For this review, take the finished solid that the model builds, in its own axes (mm). Face numbers are marked on the shaded views. A direction names the side the tool comes from. Give positions to 0.01 mm unless a question says otherwise; leave off trailing zeros. Order: outer loops, then holes, each group sorted by start corner. A loop starts at its lowest first (then second) coordinate and runs counter-clockwise, first axis right, second up. Notation, with made-up numbers: (26, 22) -> (41, 22) arc R6 ccw to (41, 27) -> close; hole circle Ø8 at (72, 78.25). An arc over 180 degrees is marked (long way). Return JSON: item names as keys, results as strings. Group by question number.
1) To check wall thickness, follow line 1 along X through (y, z) = (2, -74); line 2 along X through (y, z) = (9.3, -6); line 3 along Z through (x, y) = (73, 3.5). State the ranges of each line that lie inside material, in increasing order.
2) Add section A-A (z = -45). Give the boundary of the cut face in (x, y), then the cut area to 3 significant figures.
3) The part is to be moulded in two halves that separate along Z. For the marked faces 3, 4, 5 and 6, say which applies: released by +Z, released by -Z, zero draft, split by the parting line, or undercut.
4) Insertion check: P1, Ø7, axis at x = 25, z = -45, coming from the -Y side; P2, Ø2.5, axis at x = 105, z = -6, coming from the +Y side; P3, Ø6, axis at x = 6, z = -6, coming from the -Y side. Each pin has a flat end and moves straight along its axis. Give the tip position at first contact, or say it passes through.
5) Add section C-C (x = 69.5). Give the boundary of the cut face in (y, z), then the cut area to 3 significant figures.
6) Add section D-D (z = -59.5). Give the boundary of the cut face in (x, y).
7) Add section B-B (y = 4.25). State how many separate pieces and enclosed holes the cut face has, then the cut area to 3 significant figures.
8) For the marked faces 1 and 2, list the 3-axis set-ups (+Z, -Z, +X, -X, +Y, -Y) from which the entire face can be reached by the end or side of a thin tool; tool diameter is ignored.
from build123d import *

# Parameters (mm, degrees)
SKETCH1_W            = 110
SKETCH1_H            = 90
BOSS_EXTRUDE1_DEPTH  = 10
SHELL2_T             = -2
FILLET3_R            = 5
FILLET4_R            = 5
SKETCH5_R            = 4
BOSS_EXTRUDE12_DEPTH = 8
FILLET5_R            = 5
FILLET6_DEPTH        = 9
FILLET7_R            = 5
FILLET8_R            = 5
FILLET9_R            = 5
FILLET10_R           = 5
FILLET11_DEPTH       = 9
FILLET12_DEPTH       = 9
SKETCH6_R            = 1.6
CUT_EXTRUDE1_DEPTH   = 10
SKETCH7_R            = 4
BOSS_EXTRUDE13_DEPTH = 10
SKETCH8_R            = 1.5
CUT_EXTRUDE2_DEPTH   = 8
SKETCH9_R            = 2.75
CUT_EXTRUDE3_DEPTH   = 10
SKETCH10_R           = 2
CUT_EXTRUDE7_DEPTH   = 10
SKETCH11_R           = 2.5
CUT_EXTRUDE8_DEPTH   = 2


with BuildPart() as part:
    # Sketch1 → Boss-Extrude1 (new body)
    with BuildSketch(Plane(origin=(0, 0, 0), x_dir=(1, 0, 0), z_dir=(0, 1, 0))):
        with Locations((55, 45)):
            Rectangle(SKETCH1_W, SKETCH1_H)
    extrude(amount=BOSS_EXTRUDE1_DEPTH)

    # Shell2
    shell2_openings = [part.faces().sort_by_distance(p)[0] for p in [
        (55, 0, -45),
    ]]
    offset(amount=SHELL2_T, openings=shell2_openings, kind=Kind.INTERSECTION)

    # Fillet3
    fillet3_edges = [part.edges().sort_by_distance(p)[0] for p in [
        (0, 5, -90),
        (110, 5, -90),
        (110, 5, 0),
        (0, 5, 0),
    ]]
    fillet(fillet3_edges, radius=FILLET3_R)

    # Fillet4
    fillet4_edges = [part.edges().sort_by_distance(p)[0] for p in [
        (2, 4, -88),
        (2, 4, -2),
        (108, 4, -2),
        (108, 4, -88),
    ]]
    fillet(fillet4_edges, radius=FILLET4_R)

    # Sketch5 → Boss-Extrude12 (add)
    with BuildSketch(Plane(origin=(0, 8, 0), x_dir=(-1, 0, 0), z_dir=(0, -1, 0))):
        with Locations((-104, 6)):
            Circle(SKETCH5_R)
        with Locations((-104, 84)):
            Circle(SKETCH5_R)
        with Locations((-6, 84)):
            Circle(SKETCH5_R)
        with Locations((-6, 6)):
            Circle(SKETCH5_R)
    extrude(amount=BOSS_EXTRUDE12_DEPTH)

    # Fillet5
    # the kernel refuses this fillet: 5 mm, written as the material it adds along each edge
    with BuildSketch(Plane(origin=(107.972048604, 0, -6.472048604), x_dir=(-0.7834590295976485, 0, -0.621443439857491), z_dir=(0, 1, 0))) as fillet5_piece_1_section:
        with BuildLine():
            CenterArc((9.160403969, -3.547792862), FILLET5_R, 134.800989095, 83.620629792)
            Line((5.243108821, -6.655010061), (4.851379306, -6.965731781))
            ThreePointArc((4.851379306, -6.965731781), (-0.085536357, -0.74172022), (-0.422348831, -0.26762187))
            Line((-0.422348831, -0.26762187), (0.35232323, 0.354779286))
            ThreePointArc((0.35232323, 0.354779286), (2.818585837, -0.661765711), (5.284848444, 0.354779286))
            Line((5.284848444, 0.354779286), (5.637171673, 0))
        make_face()
    fillet5_piece_1 = extrude(amount=29.180673535, mode=Mode.PRIVATE)
    fillet5_piece_1 = split(fillet5_piece_1, bisect_by=Plane(origin=(107.972048604, 10, -6.472048604), z_dir=(0, -1, 0)), keep=Keep.TOP, mode=Mode.PRIVATE)
    add(fillet5_piece_1)

    # Fillet6: read off the stored shape, not the designer's step
    # Fillet6 outline → Fillet6 (add)
    with BuildSketch(Plane(origin=(0, 0, 0), x_dir=(1, 0, 0), z_dir=(0, 1, 0))):
        with BuildLine():
            ThreePointArc((100.02476804, 6.444444444), (98.389061423, 3.273220038), (95.05572809, 2))
            Line((95.05572809, 2), (103, 2))
            ThreePointArc((103, 2), (103.264345398, 2.006992739), (103.527951396, 2.027951396))
            ThreePointArc((103.527951396, 2.027951396), (100.866163882, 3.51422624), (100.02476804, 6.444444444))
        make_face()
    extrude(amount=FILLET6_DEPTH)

    # Fillet7
    # the kernel refuses this fillet: 5 mm, written as the material it adds along each edge
    with BuildSketch(Plane(origin=(107.972048604, 0, -83.527951396), x_dir=(0.0032991627515109216, 0, 0.9999945577477605), z_dir=(0, 1, 0))) as fillet7_piece_1_section:
        with BuildLine():
            CenterArc((8.4557736, -4.999972789), FILLET7_R, 89.810971555, 83.620629792)
            Line((3.488593561, -4.428026585), (2.991875557, -4.370831965))
            ThreePointArc((2.991875557, -4.370831965), (2.264117061, -1.804476076), (-0.060643809, -0.496308703))
            Line((-0.060643809, -0.496308703), (-0.051154492, 0.497376334))
            ThreePointArc((-0.051154492, 0.497376334), (0.52969032, 0.526206725), (8.473918995, 0.499997279))
            Line((8.473918995, 0.499997279), (8.472269414, 0))
        make_face()
    fillet7_piece_1 = extrude(amount=29.180673535, mode=Mode.PRIVATE)
    fillet7_piece_1 = split(fillet7_piece_1, bisect_by=Plane(origin=(107.972048604, 10, -83.527951396), z_dir=(0, -1, 0)), keep=Keep.TOP, mode=Mode.PRIVATE)
    add(fillet7_piece_1)

    # Fillet8
    # the kernel refuses this fillet: 5 mm, written as the material it adds along each edge
    with BuildSketch(Plane(origin=(103.527951396, 0, -87.972048604), x_dir=(-0.6214434398574978, 0, 0.783459029597643), z_dir=(0, 1, 0))) as fillet8_piece_1_section:
        with BuildLine():
            CenterArc((9.160403969, -3.547792862), FILLET8_R, 134.800989095, 83.620629792)
            Line((5.243108821, -6.655010061), (4.851379306, -6.965731781))
            ThreePointArc((4.851379306, -6.965731781), (-0.085536357, -0.74172022), (-0.422348831, -0.26762187))
            Line((-0.422348831, -0.26762187), (0.35232323, 0.354779286))
            ThreePointArc((0.35232323, 0.354779286), (2.818585837, -0.661765711), (5.284848444, 0.354779286))
            Line((5.284848444, 0.354779286), (5.637171673, 0))
        make_face()
    fillet8_piece_1 = extrude(amount=29.180673535, mode=Mode.PRIVATE)
    fillet8_piece_1 = split(fillet8_piece_1, bisect_by=Plane(origin=(103.527951396, 10, -87.972048604), z_dir=(0, -1, 0)), keep=Keep.TOP, mode=Mode.PRIVATE)
    add(fillet8_piece_1)

    # Fillet9
    # the kernel refuses this fillet: 5 mm, written as the material it adds along each edge
    with BuildSketch(Plane(origin=(6.472048604, 29.180673535, -2.027951396), x_dir=(0.9999945577477605, 0, 0.003299162751511756), z_dir=(0, -1, 0))) as fillet9_piece_1_section:
        with BuildLine():
            CenterArc((8.4557736, -4.999972789), FILLET9_R, 89.810971555, 83.620629792)
            Line((3.488593561, -4.428026585), (2.991875557, -4.370831965))
            ThreePointArc((2.991875557, -4.370831965), (2.264117061, -1.804476076), (-0.060643809, -0.496308703))
            Line((-0.060643809, -0.496308703), (-0.051154492, 0.497376334))
            ThreePointArc((-0.051154492, 0.497376334), (0.52969032, 0.526206725), (8.473918995, 0.499997279))
            Line((8.473918995, 0.499997279), (8.472269414, 0))
        make_face()
    fillet9_piece_1 = extrude(amount=29.180673535, mode=Mode.PRIVATE)
    fillet9_piece_1 = split(fillet9_piece_1, bisect_by=Plane(origin=(6.472048604, 10, -2.027951396), z_dir=(0, -1, 0)), keep=Keep.TOP, mode=Mode.PRIVATE)
    add(fillet9_piece_1)

    # Fillet10
    # the kernel refuses this fillet: 5 mm, written as the material it adds along each edge
    with BuildSketch(Plane(origin=(2.027951396, 29.180673535, -6.472048604), x_dir=(0.783459029597646, 0, -0.6214434398574942), z_dir=(0, -1, 0))) as fillet10_piece_1_section:
        with BuildLine():
            CenterArc((9.160403969, -3.547792862), FILLET10_R, 134.800989095, 83.620629792)
            Line((5.243108821, -6.655010061), (4.851379306, -6.965731781))
            ThreePointArc((4.851379306, -6.965731781), (-0.085536357, -0.74172022), (-0.422348831, -0.26762187))
            Line((-0.422348831, -0.26762187), (0.35232323, 0.354779286))
            ThreePointArc((0.35232323, 0.354779286), (2.818585837, -0.661765711), (5.284848444, 0.354779286))
            Line((5.284848444, 0.354779286), (5.637171673, 0))
        make_face()
    fillet10_piece_1 = extrude(amount=29.180673535, mode=Mode.PRIVATE)
    fillet10_piece_1 = split(fillet10_piece_1, bisect_by=Plane(origin=(2.027951396, 10, -6.472048604), z_dir=(0, -1, 0)), keep=Keep.TOP, mode=Mode.PRIVATE)
    add(fillet10_piece_1)

    # Fillet11: read off the stored shape, not the designer's step
    # Fillet11 outline → Fillet11 (add)
    with BuildSketch(Plane(origin=(0, 0, 0), x_dir=(1, 0, 0), z_dir=(0, 1, 0))):
        with BuildLine():
            ThreePointArc((2, 75.05572809), (3.273220038, 78.389061423), (6.444444444, 80.02476804))
            ThreePointArc((6.444444444, 80.02476804), (3.51422624, 80.866163882), (2.027951396, 83.527951396))
            ThreePointArc((2.027951396, 83.527951396), (2.006992739, 83.264345398), (2, 83))
            Line((2, 83), (2, 75.05572809))
        make_face()
    extrude(amount=FILLET11_DEPTH)

    # Fillet12: read off the stored shape, not the designer's step
    # Fillet12 outline → Fillet12 (add)
    with BuildSketch(Plane(origin=(0, 0, 0), x_dir=(1, 0, 0), z_dir=(0, 1, 0))):
        with BuildLine():
            ThreePointArc((9.97523196, 83.555555556), (11.610938577, 86.726779962), (14.94427191, 88))
            Line((14.94427191, 88), (7, 88))
            ThreePointArc((7, 88), (6.735654602, 87.993007261), (6.472048604, 87.972048604))
            ThreePointArc((6.472048604, 87.972048604), (9.133836118, 86.48577376), (9.97523196, 83.555555556))
        make_face()
    extrude(amount=FILLET12_DEPTH)

    # Sketch6 → Cut-Extrude1 (cut)
    with BuildSketch(Plane(origin=(0, 0, 0), x_dir=(-1, 0, 0), z_dir=(0, -1, 0))):
        with Locations(Location((-6, 6, 0), (0, 0, 90))):
            Circle(SKETCH6_R)
        with Locations(Location((-104, 84, 0), (0, 0, 90))):
            Circle(SKETCH6_R)
        with Locations(Location((-104, 6, 0), (0, 0, 90))):
            Circle(SKETCH6_R)
        with Locations(Location((-6, 84, 0), (0, 0, 90))):
            Circle(SKETCH6_R)
    extrude(amount=-CUT_EXTRUDE1_DEPTH, mode=Mode.SUBTRACT)

    # Sketch7 → Boss-Extrude13 (add)
    with BuildSketch(Plane(origin=(0, 8, 0), x_dir=(-1, 0, 0), z_dir=(0, -1, 0))):
        with Locations(Location((-95.5, 15.7, 0), (0, 0, 90))):
            Circle(SKETCH7_R)
        with Locations(Location((-95.5, 74, 0), (0, 0, 90))):
            Circle(SKETCH7_R)
        with Locations(Location((-16, 74, 0), (0, 0, 90))):
            Circle(SKETCH7_R)
        with Locations(Location((-16, 15.7, 0), (0, 0, 90))):
            Circle(SKETCH7_R)
    extrude(amount=BOSS_EXTRUDE13_DEPTH)

    # Sketch8 → Cut-Extrude2 (cut)
    with BuildSketch(Plane(origin=(0, -2, 0), x_dir=(-1, 0, 0), z_dir=(0, -1, 0))):
        with Locations(Location((-95.5, 15.7, 0), (0, 0, 90))):
            Circle(SKETCH8_R)
        with Locations(Location((-16, 15.7, 0), (0, 0, 90))):
            Circle(SKETCH8_R)
        with Locations(Location((-16, 74, 0), (0, 0, 90))):
            Circle(SKETCH8_R)
        with Locations(Location((-95.5, 74, 0), (0, 0, 90))):
            Circle(SKETCH8_R)
    extrude(amount=-CUT_EXTRUDE2_DEPTH, mode=Mode.SUBTRACT)

    # Sketch9 → Cut-Extrude3 (cut)
    with BuildSketch(Plane(origin=(0, 10, 0), x_dir=(1, 0, 0), z_dir=(0, 1, 0))):
        with Locations(Location((25, 45, 0), (0, 0, 270))):
            Circle(SKETCH9_R)
    extrude(amount=-CUT_EXTRUDE3_DEPTH, mode=Mode.SUBTRACT)

    # Sketch10 → Cut-Extrude7 (cut)
    with BuildSketch(Plane(origin=(0, 10, 0), x_dir=(1, 0, 0), z_dir=(0, 1, 0))):
        with Locations((22.25, 45)):
            Circle(SKETCH10_R)
    extrude(amount=-CUT_EXTRUDE7_DEPTH, mode=Mode.SUBTRACT)

    # Sketch11 → Cut-Extrude8 (cut)
    with BuildSketch(Plane(origin=(0, 10, 0), x_dir=(1, 0, 0), z_dir=(0, 1, 0))):
        with Locations(Location((6, 6, 0), (0, 0, 270))):
            Circle(SKETCH11_R)
        with Locations(Location((6, 84, 0), (0, 0, 270))):
            Circle(SKETCH11_R)
        with Locations(Location((104, 84, 0), (0, 0, 270))):
            Circle(SKETCH11_R)
        with Locations(Location((104, 6, 0), (0, 0, 270))):
            Circle(SKETCH11_R)
    extrude(amount=-CUT_EXTRUDE8_DEPTH, mode=Mode.SUBTRACT)


solid = part.part
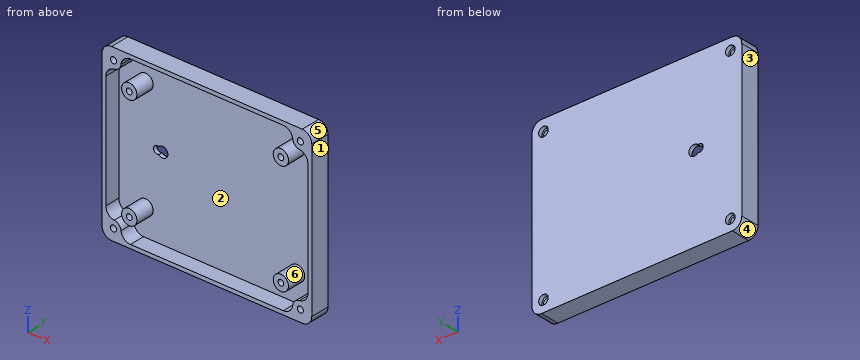
Evaluation:
{
 "1": {"line 1": "0 to 2, 12 to 14.5, 17.5 to 20, 91.5 to 94, 97 to 99.5, 108 to 110", "line 2": "0 to 3.5, 8.5 to 101.5, 106.5 to 110", "line 3": "-90 to -88, -2 to 0"},
 "2": {"outline": "(0, 0) -> (2, 0) -> (2, 8) -> (20.25, 8) -> (20.25, 10) -> (0, 10) -> close; (27.75, 8) -> (108, 8) -> (108, 0) -> (110, 0) -> (110, 10) -> (27.75, 10) -> close", "area": "237 mm^2"},
 "3": {"face 3": "zero draft", "face 4": "released by -Z", "face 5": "released by +Z", "face 6": "undercut"},
 "4": {"P1": "y = 8", "P2": "y = 8", "P3": "y = 0"},
 "5": {"outline": "(0, -90) -> (10, -90) -> (10, 0) -> (0, 0) -> (0, -2) -> (8, -2) -> (8, -88) -> (0, -88) -> close", "area": "212 mm^2"},
 "6": {"outline": "(0, 0) -> (2, 0) -> (2, 8) -> (108, 8) -> (108, 0) -> (110, 0) -> (110, 10) -> (0, 10) -> close"},
 "7": {"separate pieces": "5", "enclosed holes": "9", "area": "1,190 mm^2"},
 "8": {"face 1": "+Z, -Z, +X, +Y, -Y", "face 2": "-Y"}
}
